Answer from the drawing. Dimensions are ordinates in mm from the lowest x, y and z of the part. A direction names the side the tool comes from. Coordinates: 2 decimals unless noted, no trailing zeros. Write each loop counter-clockwise with the first axis right and the second up, starting at its lowest first coordinate (ties: lowest second). Pieces come first, ordered by that corner, then holes.
(1) Find the intervals of material crossed by probe 1 along Y at (x, z) = (12.75, 3.1); probe 2 along Y at (x, z) = (14.75, 4.15) (1 decimal); probe 3 along Y at (x, z) = (2.5, 1.5), in increasing order.
(2) Given pin 1 (1.4 mm diameter, centred on x = 14.5, z = 1.5, fed in from +Y) (1 decimal); pin 2 (6 mm diameter, centred on x = 8, y = 36, fed in from -Z); pin 3 (2.5 mm diameter, centred on x = 14.5, z = 3, fed in from -Y); pin 4 (1.4 mm diameter, centred on y = 27, z = 1.5, fed in from +X) (1 decimal), each flat-ended and moving along its own axis, determine where each tip first touches the part or whether it passes through.
(3) The mould has two halves that part along Y. Classify the marked faces 3, 4 and 5: +Y half, -Y half, draft (parallel to the pull), parting line (faces both ways), or undercut.
(4) Which of the six approach directions +Z, -Z, +X, -X, +Y, -Y give full straight-line access (tool end or side, diameter ignored) to the marked faces 1 and 2?
(5) Section B-B on y = 29 is taken. Write down the section's boundary in (x, z) (1 decimal).
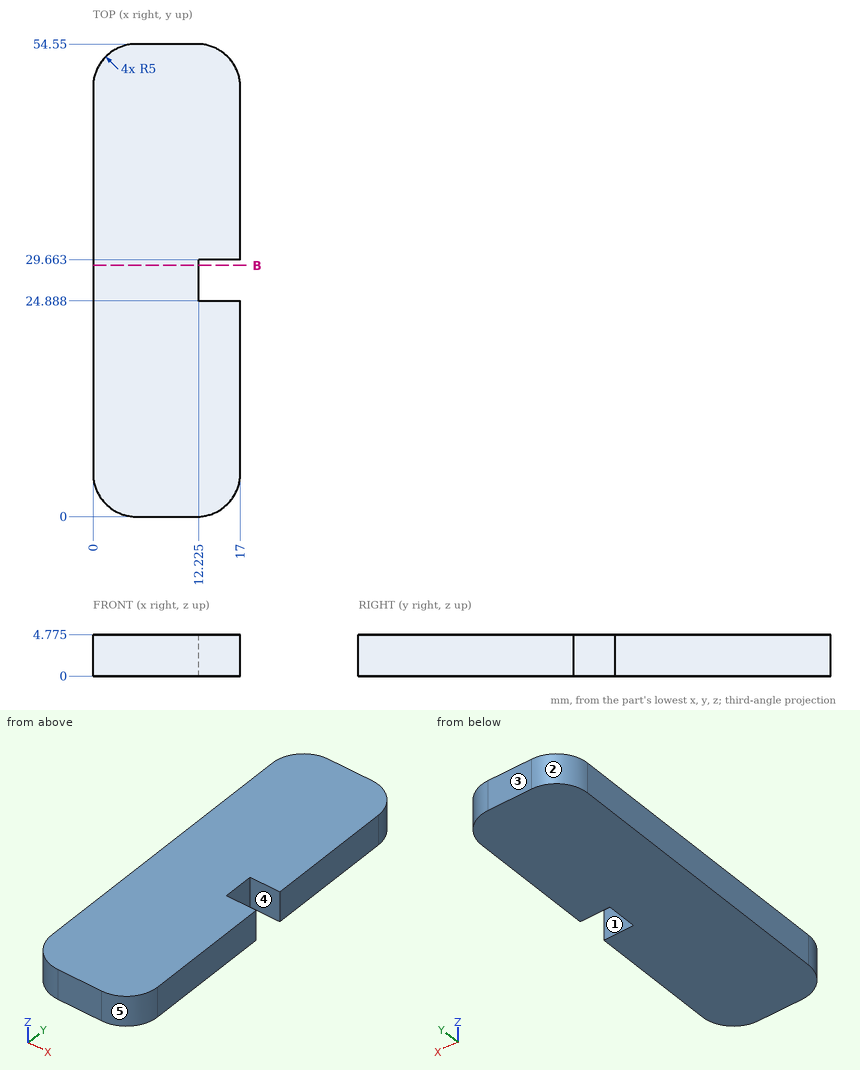
Response:
1. probe 1: y = 0.06 to 24.89, 29.66 to 54.49
1. probe 2: y = 0.8 to 24.9, 29.7 to 53.7
1. probe 3: y = 0.67 to 53.88
2. pin 1: stops at y = 54.2
2. pin 2: stops at z = 0
2. pin 3: stops at y = 0.16
2. pin 4: stops at x = 12.2
3. face 3: +Y half
3. face 4: undercut
3. face 5: -Y half
4. face 1: +Z, -Z, +X
4. face 2: +Z, -Z, -X, +Y
5. outline: (0, 0) - (12.2, 0) - (12.2, 4.8) - (0, 4.8) - close
